Here's how the part is built. I have some questions about the finished solid (model axes, mm). A direction names the side the tool comes from. Give positions to 0.01 mm unless a question says otherwise; leave off trailing zeros. Loops run counter-clockwise (first coordinate to the right, second up) from the corner with the lowest first, then second, coordinate; pieces in that order, holes last. Notation, with made-up numbers: (43.5, -34.75) -> (57.5, -34.75) arc R38 ccw to (57.5, 4.25) -> close; hole circle Ø6 at (33.25, 83.25). An arc over 180 degrees is marked (long way). Answer in a Markdown table with one row per item. Add a question column.
Item 1: If we section it at A-A (z = 4.75): Write out the boundary of the cut face in (x, y).
Item 2: Which directions (+Z, -Z, +X, -X, +Y, -Y) give clear straight access to the entire face, cutting with the end or side of a thin tool? Please do faces 5 (the face through (1, 12, 3)), 6 (the face through (-15.86, 8.65, 4.97)), 7 (the face through (-12.5, 6.5, 1.5)).
Item 3: If we section it at D-D (x = -20.75): Write out the boundary of the cut face in (y, z).
Item 4: If we section it at C-C (y = 7.25): Write out the boundary of the cut face in (x, z).
Item 5: We'd pull the mould along Y, two halves only. Please class faces 1 (the face through (-13, 4.44, 1.48)), 2 (the face through (-9.29, 10.4, 1.48)), 3 (the face through (-19.406, 10.934, 3.451)), 4 (the face through (-9.33, 4.7, 1.48)): released by +Y, released by -Y, zero draft, split by the parting line, or undercut.
Item 6: If we section it at B-B (y = 1.75): Write out the boundary of the cut face in (x, z).
Item 7: For P1, Ø9, axis at x = -7.5, y = 1.5, coming from the +Z side; P2, Ø3.5, axis at x = -6.5, z = 1, coming from the +Y side; P3, Ø2.5, axis at y = 8, z = 1.5, coming from the -X side, each with a flat end and sliding along its axis, tell me the tip position at first contact or that it passes through.
Item 8: If I drill on line 1 (Y direction, x = 0, z = 1.75); line 2 (Z direction, x = 0.75, y = 8.75); line 3 (X direction, y = -2.25, z = 2.5), over which ranges is the centre line in solid material (lowest first)?
```python
from build123d import *

# Parameters (mm, degrees)
ESQUISSE1_R          = 2.5
BASE_EXTRUSION_DEPTH = 3
BOSS_EXTRU_1_DEPTH   = 7


with BuildPart() as part:
    # Esquisse1 → Base-Extrusion (new body)
    with BuildSketch(Plane.XY):
        with BuildLine():
            Line((-10.667800722, 2.931775933), (-19.844250261, 8.864938219))
            ThreePointArc((-19.844250261, 8.864938219), (-20.280859603, 9.905812475), (-19.469453705, 10.690457238))
            Line((-19.469453705, 10.690457238), (-3.313828745, 13.446463599))
            ThreePointArc((-3.313828745, 13.446463599), (-3.022713301, 13.543930034), (-2.774883777, 13.725116223))
            Line((-2.774883777, 13.725116223), (-0.707106781, 15.792893219))
            ThreePointArc((-0.707106781, 15.792893219), (0.382683432, 16.00966597), (1, 15.085786438))
            Line((1, 15.085786438), (1, 5.766281297))
            ThreePointArc((1, 5.766281297), (1.290299171, 4.728532254), (2.076923077, 3.992040898))
            ThreePointArc((2.076923077, 3.992040898), (2.481066389, -3.75423888), (-4.486704107, -0.345667841))
            ThreePointArc((-4.486704107, -0.345667841), (-4.944162699, 0.780843297), (-5.969520458, 1.434247592))
            Line((-5.969520458, 1.434247592), (-9.231194787, 2.296710044))
            ThreePointArc((-9.231194787, 2.296710044), (-9.974591181, 2.557478226), (-10.667800722, 2.931775933))
        make_face()
        Circle(ESQUISSE1_R, mode=Mode.SUBTRACT)
        with BuildLine():
            Line((-2, 9.15321079), (-2, 5.5))
            ThreePointArc((-2, 5.5), (-2.292893219, 4.792893219), (-3, 4.5))
            Line((-3, 4.5), (-7.934127615, 4.5))
            ThreePointArc((-7.934127615, 4.5), (-9.349403144, 4.704481761), (-10.648919459, 5.301201929))
            Line((-10.648919459, 5.301201929), (-14.446834044, 7.756796926))
            ThreePointArc((-14.446834044, 7.756796926), (-14.883443387, 8.797671182), (-14.072037489, 9.582315945))
            Line((-14.072037489, 9.582315945), (-4.37665324, 11.236262526))
            ThreePointArc((-4.37665324, 11.236262526), (-3.033695989, 10.992947624), (-2.159511991, 9.944835677))
            Line((-2.159511991, 9.944835677), (-2.119182379, 9.833302751))
            ThreePointArc((-2.119182379, 9.833302751), (-2.030020908, 9.4984388), (-2, 9.15321079))
        make_face(mode=Mode.SUBTRACT)
    extrude(amount=BASE_EXTRUSION_DEPTH)

    # Esquisse2 → Boss.-Extru.1 (add)
    with BuildSketch(Plane(origin=(0, 0, 0), x_dir=(-1, 0, 0), z_dir=(0, 0, -1))):
        with BuildLine():
            Line((0.707106781, 15.792893219), (3.25, 13.25))
            Line((3.25, 13.25), (0.218577995, 10.218577995))
            ThreePointArc((0.218577995, 10.218577995), (0.056366321, 10.110191619), (-0.134975396, 10.072131386))
            Line((-0.134975396, 10.072131386), (-1, 10.072131386))
            Line((-1, 10.072131386), (-1, 15.085786438))
            ThreePointArc((-1, 15.085786438), (-0.382683432, 16.00966597), (0.707106781, 15.792893219))
        make_face()
        with BuildLine():
            Line((16.3, 11.231137936), (15.406918032, 5.995918767))
            ThreePointArc((15.406918032, 5.995918767), (20.133394575, 9.10050758), (24.105145399, 13.125833357))
            Line((24.105145399, 13.125833357), (23.004987611, 14.225991144))
            Line((23.004987611, 14.225991144), (20.200649548, 11.421653081))
            ThreePointArc((20.200649548, 11.421653081), (19.393155824, 10.930114551), (18.450112359, 10.864347833))
            Line((18.450112359, 10.864347833), (16.3, 11.231137936))
        make_face()
    extrude(amount=-BOSS_EXTRU_1_DEPTH)


solid = part.part
```
Recorded:
| question | item | result |
|---|---|---|
| 1 | outline | (-24.11, 13.13) arc R26.86 ccw to (-15.41, 6) -> (-16.3, 11.23) -> (-18.45, 10.86) arc R2 cw to (-20.2, 11.42) -> (-23, 14.23) -> close; (-3.25, 13.25) -> (-0.22, 10.22) arc R0.5 ccw to (0.13, 10.07) -> (1, 10.07) -> (1, 15.09) arc R1 ccw to (-0.71, 15.79) -> close |
| 2 | face 5 | +Z, -Z, +X, +Y |
| 2 | face 6 | +Z, +Y |
| 2 | face 7 | +Z, -Z |
| 3 | outline | (9.62, 0) -> (11.97, 0) -> (11.97, 7) -> (9.62, 7) -> close |
| 4 | outline | (-17.58, 0) -> (-13.66, 0) -> (-13.66, 3) -> (-15.62, 3) -> (-15.62, 7) -> (-17.58, 7) -> close; (-2, 0) -> (1, 0) -> (1, 3) -> (-2, 3) -> close |
| 5 | face 1 | released by -Y |
| 5 | face 2 | undercut |
| 5 | face 3 | released by +Y |
| 5 | face 4 | undercut |
| 6 | outline | (-7.16, 0) -> (-1.79, 0) -> (-1.79, 3) -> (-7.16, 3) -> close; (1.79, 0) -> (4.15, 0) -> (4.15, 3) -> (1.79, 3) -> close |
| 7 | P1 | stops at z = 3 |
| 7 | P2 | stops at y = 13.2 |
| 7 | P3 | stops at x = -20.31 |
| 8 | line 1 | y = -4.5 to -2.5, 2.5 to 16.09 |
| 8 | line 2 | z = 0 to 3 |
| 8 | line 3 | x = -3.9 to -1.09, 1.09 to 3.9 |
